Verification items for the finished model (mm, model axes). Face numbers are marked on the shaded views. A direction names the side the tool comes from. Coordinates: 2 decimals unless noted, no trailing zeros. Loops run counter-clockwise (first coordinate to the right, second up) from the corner with the lowest first, then second, coordinate; pieces in that order, holes last. Notation, with made-up numbers: (29.5, 58.5) - (86.5, 58.5) arc R16 ccw to (86.5, 70.5) - close; hole circle Ø1 at (26, 83.25). An arc over 180 degrees is marked (long way). One line per item, written item: value. Start each with the question number.
(1) Set-up check for the marked faces 1 and 2: record each of +Z, -Z, +X, -X, +Y, -Y from which the full face is reachable in a straight line by a thin tool's end or side.
(2) Gauge pin test, flat ends, axial feed: P1, Ø4, axis at x = 3.5, y = 14, coming from the -Z side; P2, Ø1.5, axis at x = 2.5, z = 7, coming from the -Y side; P3, Ø5, axis at y = 59, z = 3.5, coming from the -X side. Record the tip position at first contact, or that the pin passes through.
(3) Section check A-A (y = 7). Record the boundary of the cut face in (x, z).
(4) Thickness scan on probe 1 along Y at (x, z) = (1.75, 4.25); probe 2 along Z at (x, y) = (-2.25, 46.5); probe 3 along X at (y, z) = (46.5, 2). Record the ranges inside material, lowest first. Write a range as [from, to].
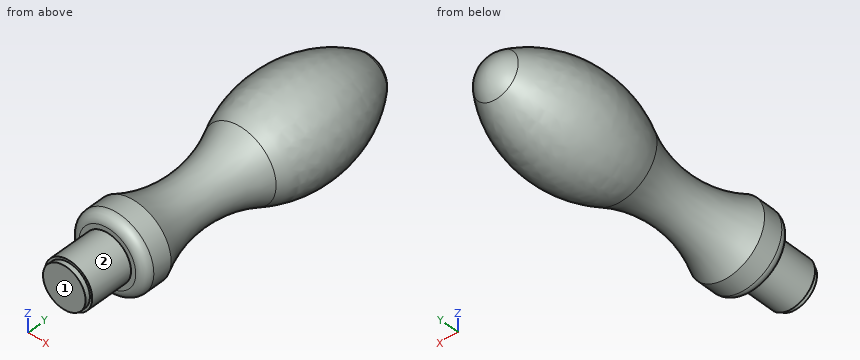
```python
from build123d import *


with BuildPart() as part:
    # Sketch1 → Revolve1 (revolve)
    with BuildSketch(Plane.XY, mode=Mode.PRIVATE) as revolve1_sk:
        with BuildLine():
            Line((0, 0), (-4.5, 0))
            Line((-4.5, 0), (-4.5, 1))
            Line((-4.5, 1), (-5, 1))
            Line((-5, 1), (-5, 10))
            Line((-5, 10), (-6, 10))
            ThreePointArc((-6, 10), (-7.414213562, 10.585786438), (-8, 12))
            Line((-8, 12), (-8, 16))
            ThreePointArc((-8, 16), (-5, 28.303061069), (-7.726981853, 40.669502823))
            ThreePointArc((-7.726981853, 40.669502823), (-10.3121962, 55.557059673), (-4.784815021, 69.620158175))
            ThreePointArc((-4.784815021, 69.620158175), (-2.671989048, 71.372194573), (0, 72))
            Line((0, 72), (0, 0))
        make_face()
    revolve(revolve1_sk.sketch.rotate(Axis((0, 0, 0), (0, 1, 0)), 270), axis=Axis((0, 0, 0), (0, 1, 0)))


solid = part.part
```
Responses:
1. face 1: +Z, -Z, +X, -X, -Y
1. face 2: -Y
2. P1: stops at z = -7.86
2. P2: stops at y = 10.12
2. P3: stops at x = -9.94
3. outline: circle Ø10 at (0, 0)
4. probe 1: y = [1, 69.86]
4. probe 2: z = [-9.49, 9.49]
4. probe 3: x = [-9.55, 9.55]
